from build123d import *

# Parameters (mm, degrees)
SKETCH1_R           = 11
SKETCH1_R_2         = 1.15
BOSS_EXTRUDE1_DEPTH = 2
SKETCH3_R           = 5
BOSS_EXTRUDE3_DEPTH = 2
SKETCH4_R           = 5
SKETCH4_R_2         = 1.5
BOSS_EXTRUDE4_DEPTH = 0.5


with BuildPart() as part:
    # Sketch1 → Boss-Extrude1 (new body)
    with BuildSketch(Plane(origin=(0, 0, 0), x_dir=(1, 0, 0), z_dir=(0, 1, 0))):
        Circle(SKETCH1_R)
        with Locations((0, -8)):
            Circle(SKETCH1_R_2, mode=Mode.SUBTRACT)
        with Locations((-6.92820323, 4)):
            Circle(SKETCH1_R_2, mode=Mode.SUBTRACT)
        with Locations((6.92820323, 4)):
            Circle(SKETCH1_R_2, mode=Mode.SUBTRACT)
        Polygon((3.175426481, 0), (1.58771324, 2.75), (-1.58771324, 2.75), (-3.175426481, 0), (-1.58771324, -2.75), (1.58771324, -2.75), align=None, mode=Mode.SUBTRACT)
    extrude(amount=BOSS_EXTRUDE1_DEPTH)

    # Sketch3 → Boss-Extrude3 (add, symmetric)
    with BuildSketch(Plane(origin=(0, 2, 0), x_dir=(1, 0, 0), z_dir=(0, 1, 0))):
        Circle(SKETCH3_R)
        Polygon((3.175426481, 0), (1.58771324, 2.75), (-1.58771324, 2.75), (-3.175426481, 0), (-1.58771324, -2.75), (1.58771324, -2.75), align=None, mode=Mode.SUBTRACT)
    extrude(amount=BOSS_EXTRUDE3_DEPTH, both=True)

    # Sketch4 → Boss-Extrude4 (add)
    with BuildSketch(Plane(origin=(0, 4, 0), x_dir=(1, 0, 0), z_dir=(0, 1, 0))):
        Circle(SKETCH4_R)
        Circle(SKETCH4_R_2, mode=Mode.SUBTRACT)
    extrude(amount=BOSS_EXTRUDE4_DEPTH)


solid = part.part
Could you check a few things on this model? Use its own coordinates, in mm. A direction names the side the tool comes from. Give positions to 0.01 mm unless a question says otherwise; leave off trailing zeros. Loops run counter-clockwise (first coordinate to the right, second up) from the corner with the lowest first, then second, coordinate; pieces in that order, holes last. Notation, with made-up numbers: M 64.5,5.25 L 70.5,5.25 A30 cw 70.5,39.25 Z; hole C 62,86.5 d3. An arc over 180 degrees is marked long. Answer as a JSON object with one key per item and string values.
Q1. For faces 1 (the cylindrical face through (0.53, 0.99, 9.02)), 2 (the flat face through (2, 2, 5)), 3 (the flat face through (1.4, 4, -1.3)), which set-ups out of +Z, -Z, +X, -X, +Y, -Y let a thin tool reach every point of the face, with its end or its side?
Values found:
{"face 1": "+Y, -Y", "face 2": "+Y", "face 3": "-Y"}
Q2. Suppose I cut it at C-C, the plane z = -4. List the corners of the cut face in (x, y) for me.
Values found:
{"outline": "M -10.25,0 L -8.08,0 L -8.08,2 L -10.25,2 Z; M -5.78,0 L 5.78,0 L 5.78,2 L 3,2 L 3,4.5 L -3,4.5 L -3,2 L -5.78,2 Z; M 8.08,0 L 10.25,0 L 10.25,2 L 8.08,2 Z"}
Q3. Suppose I cut it at B-B, the plane y = 0.9. List the corners of the cut face in (x, z) for me.
Values found:
{"outline": "C 0,0 d22; hole C -6.93,-4 d2.3; hole M -3.18,0 L -1.59,-2.75 L 1.59,-2.75 L 3.18,0 L 1.59,2.75 L -1.59,2.75 Z; hole C 0,8 d2.3; hole C 6.93,-4 d2.3"}
Q4. Suppose I cut it at D-D, the plane x = -7.5. List the corners of the cut face in (y, z) for me.
Values found:
{"outline": "M 0,-8.05 L 2,-8.05 L 2,-5 L 0,-5 Z; M 0,-3 L 2,-3 L 2,8.05 L 0,8.05 Z"}
Q5. For P1, Ø1.6, axis at x = 0.5, y = 2.5, coming from the -Z side; P2, Ø1, axis at y = 3.5, z = -1, coming from the -X side; P3, Ø5, axis at x = 0, z = 0, coming from the -Y side; P4, Ø1.5, axis at x = -2, y = 1.5, coming from the -Z side, each with a flat end and sliding along its axis, tell me the tip position at first contact or that it passes through.
Values found:
{"P1": "stops at z = -11", "P2": "stops at x = -4.97", "P3": "stops at y = 4", "P4": "stops at z = -10.93"}
Q6. If we mould it in two halves opening along Z, with no side actions, what happens to faces 4 (the flat face through (2.37, 1.972, 1.394)), 5 (the cylindrical face through (-2.38, 0.99, 10.74)), 6 (the flat face through (-1.2, 4.5, -1.2))? For each: pulls with the +Z half, pulls with the -Z half, needs draft (parallel to the pull), parting line crosses it, or undercut.
Values found:
{"face 4": "undercut", "face 5": "parting line crosses it", "face 6": "needs draft"}
Q7. If I drill on probe 1 along Z at (x, y) = (0, 1.05); probe 2 along X at (y, z) = (1, -4); probe 3 along Z at (x, y) = (0, 4.3), over which ranges is the centre line in solid material (lowest first)? Write a range as [from, to].
Values found:
{"probe 1": "z = [-11, -2.75], [2.75, 6.85], [9.15, 11]", "probe 2": "x = [-10.25, -8.08], [-5.78, 5.78], [8.08, 10.25]", "probe 3": "z = [-5, -1.5], [1.5, 5]"}
Q8. Suppose I cut it at A-A, the plane x = 0. List the corners of the cut face in (y, z) for me, plus the area to 3 significant figures.
Values found:
{"outline": "M 0,-11 L 2,-11 L 2,-5 L 4.5,-5 L 4.5,-1.5 L 4,-1.5 L 4,-2.75 L 0,-2.75 Z; M 0,2.75 L 4,2.75 L 4,1.5 L 4.5,1.5 L 4.5,5 L 2,5 L 2,6.85 L 0,6.85 Z; M 0,9.15 L 2,9.15 L 2,11 L 0,11 Z", "area": "40.9 mm²"}
